Verification items for this drawing (mm, ordinates from the low corner). A direction names the side the tool comes from. Round coordinates to 2 decimals unless told otherwise and drop trailing zeros. Loops run counter-clockwise (first coordinate to the right, second up) from the corner with the lowest first, then second, coordinate; pieces in that order, holes last. Notation, with made-up numbers: M -7.5,77.5 L -2.5,77.5 A23 cw -2.5,85.5 Z; hole C -21,-11 d8. An arc over 180 degrees is marked long. Write item = value, one per line.
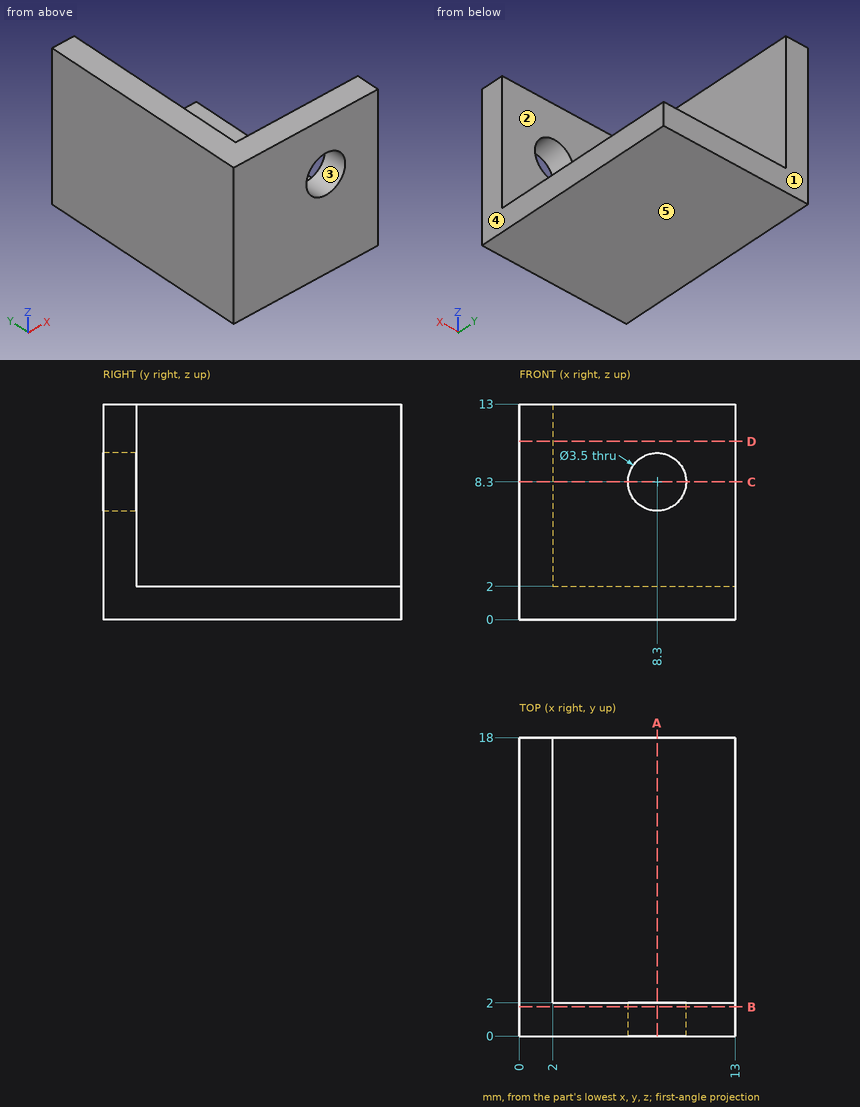
(1) Sectioned sample at B-B on y = 1.75. Record the cut outline in (x, z), then the cut area to 3 significant figures.
Result set:
outline = M 0,0 L 13,0 L 13,13 L 0,13 Z; hole C 8.3,8.3 d3.5
area = 159 mm2
(2) Sectioned sample at D-D on z = 10.75. Record the cut outline in (x, y), then the cut area to 3 significant figures.
Result set:
outline = M 0,0 L 13,0 L 13,2 L 2,2 L 2,18 L 0,18 Z
area = 58.0 mm2
(3) Depth check by flat-ended pin: pin 1 Ø1.5 at (y, z) = (11, 11.5) entering from +X; pin 2 Ø3 at (x, z) = (8.3, 8.3) entering from -Y; pin 3 Ø3.5 at (x, y) = (7, 7) entering from +Z; pin 4 Ø1.5 at (x, z) = (8.5, 7) entering from +Y. Enter the tip coordinate at first touch or a pass-through.
Result set:
pin_1 = 2
pin_2 = through
pin_3 = 2
pin_4 = 2
(4) Tool access check on the marked faces 1 and 2. Record the directions out of +Z, -Z, +X, -X, +Y, -Y that give a thin tool (end or side, any length) a straight path to the whole face; none if there is none.
Result set:
face_1 = +Z, -Z, +X, -X, +Y
face_2 = +Z, +X, +Y
(5) Sectioned sample at C-C on z = 8.3. Record the cut outline in (x, y).
Result set:
outline = M 0,0 L 6.55,0 L 6.55,2 L 2,2 L 2,18 L 0,18 Z; M 10.05,0 L 13,0 L 13,2 L 10.05,2 Z
(6) Material ranges on line 1 along X through (y, z) = (1.15, 8.3); line 2 along Z through (x, y) = (4.5, 13.75), recorded low to high. Write a range as from..to.
Result set:
line_1 = 0..6.55, 10.05..13
line_2 = 0..2
(7) Release check for a two-part mould opening along X. For the marked faces 3, 4 and 5 record: released by +X, released by -X, zero draft, split by the parting line, or undercut.
Result set:
face_3 = undercut
face_4 = released by +X
face_5 = zero draft
(8) Sectioned sample at A-A on x = 8.3. Record the cut outline in (y, z).
Result set:
outline = M 0,0 L 18,0 L 18,2 L 2,2 L 2,6.55 L 0,6.55 Z; M 0,10.05 L 2,10.05 L 2,13 L 0,13 Z
